Design review of the part built by this model. Coordinates are the model's own, in mm. Face numbers are marked on the shaded views. A direction names the side the tool comes from. Give positions to 0.01 mm unless a question says otherwise; leave off trailing zeros. Loops run counter-clockwise (first coordinate to the right, second up) from the corner with the lowest first, then second, coordinate; pieces in that order, holes last.
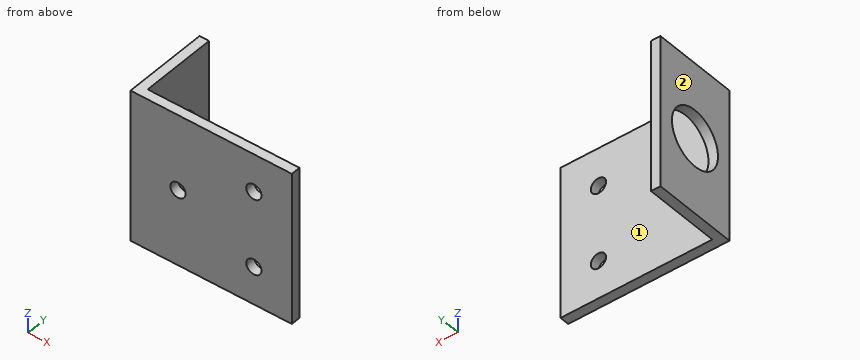
from build123d import *

# Parameters (mm, degrees)
BOSS_EXTRUDE1_DEPTH = 50.8
SKETCH2_R           = 9.525
SKETCH2_W           = 50.8
SKETCH2_H           = 22.225
CUT_EXTRUDE1_DEPTH  = 50.8
SKETCH3_R           = 2.5527
CUT_EXTRUDE2_DEPTH  = 50.8


with BuildPart() as part:
    # Sketch1 → Boss-Extrude1 (new body)
    with BuildSketch(Plane.XY):
        Polygon((3.175, 50.8), (0, 50.8), (0, 0), (3.175, 0), (53.975, 0), (53.975, 3.175), (3.175, 3.175), align=None)
    extrude(amount=BOSS_EXTRUDE1_DEPTH)

    # Sketch2 → Cut-Extrude1 (cut)
    with BuildSketch(Plane.ZY):
        with Locations((25.4, 14.2875)):
            Circle(SKETCH2_R)
        with Locations((25.4, 39.6875)):
            Rectangle(SKETCH2_W, SKETCH2_H)
    extrude(amount=-CUT_EXTRUDE1_DEPTH, mode=Mode.SUBTRACT)

    # Sketch3 → Cut-Extrude2 (cut)
    with BuildSketch(Plane(origin=(0, 0, 0), x_dir=(-1, 0, 0), z_dir=(0, -1, 0))):
        with Locations((-15.875, -25.4)):
            Circle(SKETCH3_R)
        with Locations((-41.275, -38.1)):
            Circle(SKETCH3_R)
        with Locations((-41.275, -12.7)):
            Circle(SKETCH3_R)
    extrude(amount=-CUT_EXTRUDE2_DEPTH, mode=Mode.SUBTRACT)


solid = part.part
Q1. Insertion check: pin 1 (1 mm diameter, centred on y = 7.5, z = 11.5, fed in from +X) (3 decimals); pin 2 (8 mm diameter, centred on x = 41.275, z = 12.7, fed in from +Y) (3 decimals); pin 3 (10 mm diameter, centred on y = 7.5, z = 45, fed in from +X) (3 decimals). Each pin has a flat end and moves straight along its axis. Give the tip position at first contact, or say it passes through.
Results:
pin 1: stops at x = 3.175
pin 2: stops at y = 3.175
pin 3: stops at x = 53.975
Q2. Take a section at B-B (x = 42). Give the boundary of the cut face in (y, z) (3 decimals).
Results:
outline: (0, 0) - (3.175, 0) - (3.175, 10.252) - (0, 10.252) - close; (0, 15.148) - (3.175, 15.148) - (3.175, 35.652) - (0, 35.652) - close; (0, 40.548) - (3.175, 40.548) - (3.175, 50.8) - (0, 50.8) - close
Q3. Take a section at D-D (z = 25.4). Give the boundary of the cut face in (x, y) (1 decimal), plus the area to 3 significant figures.
Results:
outline: (0, 0) - (13.3, 0) - (13.3, 3.2) - (3.2, 3.2) - (3.2, 4.8) - (0, 4.8) - close; (0, 23.8) - (3.2, 23.8) - (3.2, 28.6) - (0, 28.6) - close; (18.4, 0) - (54, 0) - (54, 3.2) - (18.4, 3.2) - close
area: 175 mm2
Q4. Wall thickness on line 1 (Y direction, x = 2.1, z = 25.4) (1 decimal); line 2 (X direction, y = 0.9, z = 38.1) (3 decimals); line 3 (X direction, y = 24, z = 40.5) (3 decimals): over which ranges is each line inside the solid? List them lowest first.
Results:
line 1: y = 0 to 4.8, 23.8 to 28.6
line 2: x = 0 to 38.722, 43.828 to 53.975
line 3: x = 0 to 3.175
Q5. Take a section at A-A (z = 38.1). Give the boundary of the cut face in (x, y) (3 decimals), plus the area to 3 significant figures.
Results:
outline: (0, 0) - (38.722, 0) - (38.722, 3.175) - (3.175, 3.175) - (3.175, 28.575) - (0, 28.575) - close; (43.828, 0) - (53.975, 0) - (53.975, 3.175) - (43.828, 3.175) - close
area: 236 mm2
Q6. Tool access review of the marked faces 1 and 2: name each direction out of +Z, -Z, +X, -X, +Y, -Y from which nothing blocks a thin tool from reaching the whole face with its end or side.
Results:
face 1: +Z, -Z, +X, +Y
face 2: +Z, -Z, -X, +Y, -Y
Q7. Take a section at C-C (y = 17.25). Give the boundary of the cut face in (x, z) (3 decimals), plus the area to 3 significant figures.
Results:
outline: (0, 0) - (3.175, 0) - (3.175, 16.347) - (0, 16.347) - close; (0, 34.453) - (3.175, 34.453) - (3.175, 50.8) - (0, 50.8) - close
area: 104 mm2
